Geometry: final body of the model. Coordinates: model frame, mm. A direction names the side the tool comes from. Coordinates: 2 decimals unless noted, no trailing zeros. Loops run counter-clockwise (first coordinate to the right, second up) from the corner with the lowest first, then second, coordinate; pieces in that order, holes last. Notation, with made-up numbers: (-25, 26.25) -> (23, 26.25) arc R19 ccw to (23, 57.25) -> close; hole circle Ø7 at (40, -3). An arc over 180 degrees is marked (long way). One line per item, written item: value. Start each with the question number.
from build123d import *

# Parameters (mm, degrees)
SKETCH1_R           = 315
SKETCH1_R_2         = 217.5
SKETCH1_R_3         = 6
SKETCH1_R_4         = 2
BOSS_EXTRUDE1_DEPTH = 0.75


with BuildPart() as part:
    # Sketch1 → Boss-Extrude1 (new, symmetric)
    with BuildSketch(Plane(origin=(0, 0, 0), x_dir=(1, 0, 0), z_dir=(0, 1, 0))):
        with Locations(Location((0, 0, 0), (0, 0, 270))):
            Circle(SKETCH1_R)
        with Locations(Location((0, 0, 0), (0, 0, 270))):
            Circle(SKETCH1_R_2, mode=Mode.SUBTRACT)
        with Locations(Location((0, 240, 0), (0, 0, 270))):
            Circle(SKETCH1_R_3, mode=Mode.SUBTRACT)
        with Locations(Location((169.705627485, 169.705627485, 0), (0, 0, 270))):
            Circle(SKETCH1_R_3, mode=Mode.SUBTRACT)
        with Locations(Location((240, 0, 0), (0, 0, 270))):
            Circle(SKETCH1_R_3, mode=Mode.SUBTRACT)
        with Locations(Location((169.705627485, -169.705627485, 0), (0, 0, 270))):
            Circle(SKETCH1_R_3, mode=Mode.SUBTRACT)
        with Locations(Location((0, -240, 0), (0, 0, 270))):
            Circle(SKETCH1_R_3, mode=Mode.SUBTRACT)
        with Locations(Location((-169.705627485, -169.705627485, 0), (0, 0, 270))):
            Circle(SKETCH1_R_3, mode=Mode.SUBTRACT)
        with Locations(Location((-240, 0, 0), (0, 0, 270))):
            Circle(SKETCH1_R_3, mode=Mode.SUBTRACT)
        with Locations(Location((-169.705627485, 169.705627485, 0), (0, 0, 270))):
            Circle(SKETCH1_R_3, mode=Mode.SUBTRACT)
        with Locations(Location((-231.822198309, 62.116570825, 0), (0, 0, 270))):
            Circle(SKETCH1_R_4, mode=Mode.SUBTRACT)
        with Locations(Location((-207.846062834, 120.000258819, 0), (0, 0, 270))):
            Circle(SKETCH1_R_4, mode=Mode.SUBTRACT)
        with Locations(Location((-119.999707107, 207.846804015, 0), (0, 0, 270))):
            Circle(SKETCH1_R_4, mode=Mode.SUBTRACT)
        with Locations(Location((-62.116070825, 231.823064335, 0), (0, 0, 270))):
            Circle(SKETCH1_R_4, mode=Mode.SUBTRACT)
        with Locations(Location((62.117570825, 231.823198309, 0), (0, 0, 270))):
            Circle(SKETCH1_R_4, mode=Mode.SUBTRACT)
        with Locations(Location((120.001258819, 207.847062834, 0), (0, 0, 270))):
            Circle(SKETCH1_R_4, mode=Mode.SUBTRACT)
        with Locations(Location((207.847804015, 120.000707107, 0), (0, 0, 270))):
            Circle(SKETCH1_R_4, mode=Mode.SUBTRACT)
        with Locations(Location((231.824064335, 62.117070825, 0), (0, 0, 270))):
            Circle(SKETCH1_R_4, mode=Mode.SUBTRACT)
        with Locations(Location((231.824198309, -62.116570825, 0), (0, 0, 270))):
            Circle(SKETCH1_R_4, mode=Mode.SUBTRACT)
        with Locations(Location((207.848062834, -120.000258819, 0), (0, 0, 270))):
            Circle(SKETCH1_R_4, mode=Mode.SUBTRACT)
        with Locations(Location((120.001707107, -207.846804015, 0), (0, 0, 270))):
            Circle(SKETCH1_R_4, mode=Mode.SUBTRACT)
        with Locations(Location((62.118070825, -231.823064335, 0), (0, 0, 270))):
            Circle(SKETCH1_R_4, mode=Mode.SUBTRACT)
        with Locations(Location((-62.115570825, -231.823198309, 0), (0, 0, 270))):
            Circle(SKETCH1_R_4, mode=Mode.SUBTRACT)
        with Locations(Location((-119.999258819, -207.847062834, 0), (0, 0, 270))):
            Circle(SKETCH1_R_4, mode=Mode.SUBTRACT)
        with Locations(Location((-207.845804015, -120.000707107, 0), (0, 0, 270))):
            Circle(SKETCH1_R_4, mode=Mode.SUBTRACT)
        with Locations(Location((-231.822064335, -62.117070825, 0), (0, 0, 270))):
            Circle(SKETCH1_R_4, mode=Mode.SUBTRACT)
        with Locations(Location((-289.777747887, 77.645713531, 0), (0, 0, 270))):
            Circle(SKETCH1_R_4, mode=Mode.SUBTRACT)
        with Locations(Location((-259.807621135, 150, 0), (0, 0, 270))):
            Circle(SKETCH1_R_4, mode=Mode.SUBTRACT)
        with Locations(Location((-212.132034356, 212.132034356, 0), (0, 0, 270))):
            Circle(SKETCH1_R_4, mode=Mode.SUBTRACT)
        with Locations(Location((-150, 259.807621135, 0), (0, 0, 270))):
            Circle(SKETCH1_R_4, mode=Mode.SUBTRACT)
        with Locations(Location((-77.645713531, 289.777747887, 0), (0, 0, 270))):
            Circle(SKETCH1_R_4, mode=Mode.SUBTRACT)
        with Locations(Location((0, 300, 0), (0, 0, 270))):
            Circle(SKETCH1_R_4, mode=Mode.SUBTRACT)
        with Locations(Location((77.645713531, 289.777747887, 0), (0, 0, 270))):
            Circle(SKETCH1_R_4, mode=Mode.SUBTRACT)
        with Locations(Location((150, 259.807621135, 0), (0, 0, 270))):
            Circle(SKETCH1_R_4, mode=Mode.SUBTRACT)
        with Locations(Location((212.132034356, 212.132034356, 0), (0, 0, 270))):
            Circle(SKETCH1_R_4, mode=Mode.SUBTRACT)
        with Locations(Location((259.807621135, 150, 0), (0, 0, 270))):
            Circle(SKETCH1_R_4, mode=Mode.SUBTRACT)
        with Locations(Location((289.777747887, 77.645713531, 0), (0, 0, 270))):
            Circle(SKETCH1_R_4, mode=Mode.SUBTRACT)
        with Locations(Location((300, 0, 0), (0, 0, 270))):
            Circle(SKETCH1_R_4, mode=Mode.SUBTRACT)
        with Locations(Location((289.777747887, -77.645713531, 0), (0, 0, 270))):
            Circle(SKETCH1_R_4, mode=Mode.SUBTRACT)
        with Locations(Location((259.807621135, -150, 0), (0, 0, 270))):
            Circle(SKETCH1_R_4, mode=Mode.SUBTRACT)
        with Locations(Location((212.132034356, -212.132034356, 0), (0, 0, 270))):
            Circle(SKETCH1_R_4, mode=Mode.SUBTRACT)
        with Locations(Location((150, -259.807621135, 0), (0, 0, 270))):
            Circle(SKETCH1_R_4, mode=Mode.SUBTRACT)
        with Locations(Location((77.645713531, -289.777747887, 0), (0, 0, 270))):
            Circle(SKETCH1_R_4, mode=Mode.SUBTRACT)
        with Locations(Location((0, -300, 0), (0, 0, 270))):
            Circle(SKETCH1_R_4, mode=Mode.SUBTRACT)
        with Locations(Location((-77.645713531, -289.777747887, 0), (0, 0, 270))):
            Circle(SKETCH1_R_4, mode=Mode.SUBTRACT)
        with Locations(Location((-150, -259.807621135, 0), (0, 0, 270))):
            Circle(SKETCH1_R_4, mode=Mode.SUBTRACT)
        with Locations(Location((-212.132034356, -212.132034356, 0), (0, 0, 270))):
            Circle(SKETCH1_R_4, mode=Mode.SUBTRACT)
        with Locations(Location((-259.807621135, -150, 0), (0, 0, 270))):
            Circle(SKETCH1_R_4, mode=Mode.SUBTRACT)
        with Locations(Location((-289.777747887, -77.645713531, 0), (0, 0, 270))):
            Circle(SKETCH1_R_4, mode=Mode.SUBTRACT)
        with Locations(Location((-300, 0, 0), (0, 0, 270))):
            Circle(SKETCH1_R_4, mode=Mode.SUBTRACT)
        Polygon((-53.651203475, 288.339293829), (-27.904233688, 291.957794454), (-22.894002053, 256.308143979), (-48.64097184, 252.689643354), align=None, mode=Mode.SUBTRACT)
        with BuildLine():
            Line((-19.708603347, 281.846158847), (-18.659856727, 266.848383445))
            ThreePointArc((-18.659856727, 266.848383445), (46.450887526, 263.436073931), (108.802052023, 244.373409919))
            Line((108.802052023, 244.373409919), (114.917092776, 258.108016324))
            ThreePointArc((114.917092776, 258.108016324), (49.061583418, 278.242066078), (-19.708603347, 281.846158847))
        make_face(mode=Mode.SUBTRACT)
        with BuildLine():
            Line((231.661795512, 133.75), (244.681966494, 141.267199221))
            ThreePointArc((244.681966494, 141.267199221), (203.238237764, 196.26488482), (149.720420543, 239.602758697))
            Line((149.720420543, 239.602758697), (141.753403182, 226.852865722))
            ThreePointArc((141.753403182, 226.852865722), (192.423396591, 185.821114098), (231.661795512, 133.75))
        make_face(mode=Mode.SUBTRACT)
        with BuildLine():
            Line((266.034607011, -27.961363924), (280.986645445, -29.532886489))
            ThreePointArc((280.986645445, -29.532886489), (279.784793098, 39.321188359), (261.961332595, 105.839248523))
            Line((261.961332595, 105.839248523), (248.021681097, 100.207263739))
            ThreePointArc((248.021681097, 100.207263739), (264.896708388, 37.228804507), (266.034607011, -27.961363924))
        make_face(mode=Mode.SUBTRACT)
        with BuildLine():
            Line((198.791240815, -178.992437201), (209.963976221, -189.052413347))
            ThreePointArc((209.963976221, -189.052413347), (249.463067004, -132.641865577), (274.141919334, -68.351257243))
            Line((274.141919334, -68.351257243), (259.554106779, -64.714107073))
            ThreePointArc((259.554106779, -64.714107073), (236.18848109, -125.583643045), (198.791240815, -178.992437201))
        make_face(mode=Mode.SUBTRACT)
        with BuildLine():
            Line((55.616377294, -261.654483196), (58.742204494, -276.360343961))
            ThreePointArc((58.742204494, -276.360343961), (123.854928252, -253.940235194), (181.609610629, -216.433905916))
            Line((181.609610629, -216.433905916), (171.945685591, -204.916888534))
            ThreePointArc((171.945685591, -204.916888534), (117.264281766, -240.427407385), (55.616377294, -261.654483196))
        make_face(mode=Mode.SUBTRACT)
        with BuildLine():
            Line((-108.802052023, -244.373409919), (-114.917092776, -258.108016324))
            ThreePointArc((-114.917092776, -258.108016324), (-49.061583418, -278.242066078), (19.708603347, -281.846158847))
            Line((19.708603347, -281.846158847), (18.659856727, -266.848383445))
            ThreePointArc((18.659856727, -266.848383445), (-46.450887526, -263.436073931), (-108.802052023, -244.373409919))
        make_face(mode=Mode.SUBTRACT)
        with BuildLine():
            Line((-231.661795512, -133.75), (-244.681966494, -141.267199221))
            ThreePointArc((-244.681966494, -141.267199221), (-203.238237764, -196.26488482), (-149.720420543, -239.602758697))
            Line((-149.720420543, -239.602758697), (-141.753403182, -226.852865722))
            ThreePointArc((-141.753403182, -226.852865722), (-192.423396591, -185.821114098), (-231.661795512, -133.75))
        make_face(mode=Mode.SUBTRACT)
        with BuildLine():
            Line((-266.034607011, 27.961363924), (-280.986645445, 29.532886489))
            ThreePointArc((-280.986645445, 29.532886489), (-279.784793098, -39.321188359), (-261.961332595, -105.839248523))
            Line((-261.961332595, -105.839248523), (-248.021681097, -100.207263739))
            ThreePointArc((-248.021681097, -100.207263739), (-264.896708388, -37.228804507), (-266.034607011, 27.961363924))
        make_face(mode=Mode.SUBTRACT)
        with BuildLine():
            Line((-198.791240815, 178.992437201), (-209.963976221, 189.052413347))
            ThreePointArc((-209.963976221, 189.052413347), (-249.463067004, 132.641865577), (-274.141919334, 68.351257243))
            Line((-274.141919334, 68.351257243), (-259.554106779, 64.714107073))
            ThreePointArc((-259.554106779, 64.714107073), (-236.18848109, 125.583643045), (-198.791240815, 178.992437201))
        make_face(mode=Mode.SUBTRACT)
        with BuildLine():
            Line((-55.616377294, 261.654483196), (-58.742204494, 276.360343961))
            ThreePointArc((-58.742204494, 276.360343961), (-123.854928252, 253.940235194), (-181.609610629, 216.433905916))
            Line((-181.609610629, 216.433905916), (-171.945685591, 204.916888534))
            ThreePointArc((-171.945685591, 204.916888534), (-117.264281766, 240.427407385), (-55.616377294, 261.654483196))
        make_face(mode=Mode.SUBTRACT)
    extrude(amount=BOSS_EXTRUDE1_DEPTH, both=True)


solid = part.part
1. Section A-A on x = 87. Return the cut outline in (y, z).
2. Section B-B on y = 0.15. Count the separate pieces of the cut face and the enclosed holes in it, plus the area to 3 significant figures.
3. Pin query (flat end, axial travel): pin 1 Ø5 at (x, z) = (-62.12, -231.82) entering from -Y. Return the tip coordinate at first contact, or that it passes through.
4. Line query: L1, parallel to Z at x = 149, y = -0.15; L2, parallel to Z at x = -141.5, y = -0.3; L3, parallel to X at y = -0.5, z = -97. Output: solid intervals per line, ascending. Write a range as [from, to].
5. Set-up query: faces 5 (the face through (214, -0.75, 66)), 6 (the face through (191.787, 0.01, -186.478)). Return all of +Z, -Z, +X, -X, +Y, -Y with unobstructed straight access to the full face (end or side cutting, diameter ignored); none if empty.
6. Draft query along Z for faces 1 (the face through (-307.51, 0.01, -68.29)), 2 (the face through (45.5, 0, -263.6)), 3 (the face through (214, 0.75, 66)), 4 (the face through (-45.5, 0, 263.6)). Return one class per face: released by +Z, released by -Z, zero draft, split by the parting line, or undercut.
Checks:
1. outline: (-0.75, -302.75) -> (0.75, -302.75) -> (0.75, -268.81) -> (-0.75, -268.81) -> close; (-0.75, -252.96) -> (0.75, -252.96) -> (0.75, -199.34) -> (-0.75, -199.34) -> close; (-0.75, 199.34) -> (0.75, 199.34) -> (0.75, 252.96) -> (-0.75, 252.96) -> close; (-0.75, 268.81) -> (0.75, 268.81) -> (0.75, 302.75) -> (-0.75, 302.75) -> close
2. separate pieces: 1
2. enclosed holes: 60
2. area: 141,000 mm²
3. pin 1: y = -0.75
4. L1: [-277.53, -261.54], [-258.08, -238.45], [-222.16, -158.45], [158.45, 222.16], [240.05, 258.08], [261.54, 277.53]
4. L2: [-281.43, -244.55], [-227.01, -165.18], [165.18, 281.43]
4. L3: [-299.69, -265.36], [-249.29, -194.67], [194.67, 249.29], [265.36, 299.69]
5. face 5: +Z, -Z, +X, -X, -Y
5. face 6: +Y, -Y
6. face 1: split by the parting line
6. face 2: undercut
6. face 3: zero draft
6. face 4: undercut
